Autodesk Fusion 360 part; units mm, degrees
sketch "Esquisse1" plane through (0, 0, 0) normal (0, 1, 0) x (1, 0, 0)
  line L0 (0, 0) -> (350, 0)
  line L1 (350, 0) -> (350, -350)
  line L2 (350, -350) -> (0, -350)
  line L3 (0, -350) -> (0, 0)
  dimension "d1" = 350
  dimension "d2" = 350
extrude "Extrusion1" add sketch "Esquisse1" along normal blind 350
sketch "Esquisse2" plane through (0, 0, 0) normal (0, 0, 1) x (1, 0, 0)
shell "Coque1" thickness 30 removed faces 2 at (116.6667, 116.6667, 0) at (233.3333, 116.6667, 350)
Build history of the part. All positions in model axes, mm. A direction names the side the tool comes from. Round coordinates to 2 decimals unless told otherwise and drop trailing zeros. Write each loop counter-clockwise with the first axis right and the second up, starting at its lowest first coordinate (ties: lowest second). Pieces come first, ordered by that corner, then holes. Notation, with made-up numbers: M 79,-8 L 114,-8 A31 ccw 114,27 Z; hole C 19,-4 d6. An arc over 180 degrees is marked long. Answer as a JSON object with one key per item and string values. Group by question number.
(1) Drill centre line: L1, parallel to Y at x = 150, z = 253. Where is it in solid material? Low to high.
(2) Mould opens along X. For faces 1 (the flat face through (22, 173, 350)), 2 (the flat face through (350, 173, 173)), 3 (the flat face through (320, 173, 173)) say: pulls with the +X half, pulls with the -X half, needs draft (parallel to the pull), parting line crosses it, or undercut.
(3) Cut at C-C (z = 175). Give the cut face in (x, y).
(4) Which spindle directions (+Z, -Z, +X, -X, +Y, -Y) get a long thin tool onto all of the face, cutting with end or side? Do faces 4 (the flat face through (30, 173, 177)), 5 (the flat face through (0, 173, 177)). Say none if no direction does.
(5) Cut at A-A (x = 44.5). Give the cut face in (y, z), and give its area (3 significant figures).
Responses:
{
 "1": {"L1": "y = 0 to 30, 320 to 350"},
 "2": {"face 1": "needs draft", "face 2": "pulls with the +X half", "face 3": "undercut"},
 "3": {"outline": "M 0,0 L 350,0 L 350,350 L 0,350 Z; hole M 30,30 L 320,30 L 320,320 L 30,320 Z"},
 "4": {"face 4": "+Z, -Z", "face 5": "+Z, -Z, -X, +Y, -Y"},
 "5": {"outline": "M 0,0 L 30,0 L 30,350 L 0,350 Z; M 320,0 L 350,0 L 350,350 L 320,350 Z", "area": "21,000 mm2"}
}
